CAD build for the part. Positions are in the model's coordinates, mm. A direction names the side the tool comes from. Round coordinates to 2 decimals unless told otherwise and drop trailing zeros. Loops run counter-clockwise (first coordinate to the right, second up) from the corner with the lowest first, then second, coordinate; pieces in that order, holes last. Notation, with made-up numbers: (49, 59) - (67, 59) arc R18 cw to (67, 77) - close; hole circle Ø1 at (8, 67). An arc over 180 degrees is marked (long way). One line per question, with ' | ' between items.
```python
from build123d import *

# Parameters (mm, degrees)
SKETCH_1_W          = 10
SKETCH_1_H          = 10
EXTRUDE_1_DEPTH     = 45
SKETCH_2_W          = 3
SKETCH_2_H          = 5
CUT_EXTRUDE_1_DEPTH = 7
CUT_EXTRUDE_2_REACH = 49.17
SKETCH_3_R          = 1.75


with BuildPart() as part:
    # 草图1 → 凸台-拉伸1 (new body)
    with BuildSketch(Plane.XY):
        with Locations((5, -5)):
            Rectangle(SKETCH_1_W, SKETCH_1_H)
    extrude(amount=EXTRUDE_1_DEPTH)

    # 草图2 → 切除-拉伸1 (cut)
    with BuildSketch(Plane(origin=(0, 0, 0), x_dir=(-1, 0, 0), z_dir=(0, 0, -1))):
        with Locations((-5, -5)):
            Rectangle(SKETCH_2_W, SKETCH_2_H)
    extrude(amount=-CUT_EXTRUDE_1_DEPTH, mode=Mode.SUBTRACT)

    # 草图3 → 切除-拉伸2 (cut, up to next)
    with BuildSketch(Plane(origin=(10, 0, 0), x_dir=(0, 0, -1), z_dir=(1, 0, 0)), mode=Mode.PRIVATE) as cut_extrude_2_sk1:
        with Locations(Location((-3.5, -5, 0), (0, 0, 90))):
            Circle(SKETCH_3_R)
    cut_extrude_2_tool1 = extrude(cut_extrude_2_sk1.sketch, amount=-CUT_EXTRUDE_2_REACH, mode=Mode.PRIVATE) & part.part
    add(cut_extrude_2_tool1.solids().sort_by_distance((10, -5, 3.5))[0], mode=Mode.SUBTRACT)


solid = part.part
```
(1) Drop a flat-ended pin along its axis: P1, Ø1.5, axis at x = 4.5, y = -5, coming from the -Z side. Give the stop position or say it passes through.
Results found:
P1: stops at z = 7
(2) Probe L1, parallel to Z at x = 8.75, y = -5; L2, parallel to Z at x = 4.5, y = -4.75; L3, parallel to Z at x = 7.5, y = -4. List the from-to ranges inside material, lowest first.
Results found:
L1: z = 0 to 1.75, 5.25 to 45 | L2: z = 7 to 45 | L3: z = 0 to 2.06, 4.94 to 45
(3) Tool access for faces 1 (the face through (5, -5, 7)), 2 (the face through (5, -10, 22)): list every direction of +Z, -Z, +X, -X, +Y, -Y with a clear straight run to the whole face (end or side of a thin tool).
Results found:
face 1: -Z | face 2: +Z, -Z, +X, -X, -Y
(4) Cut at A-A, the plane y = -5. Write the cut outline in (x, z), then the cut area to 3 significant figures.
Results found:
outline: (0, 0) - (3.5, 0) - (3.5, 7) - (6.5, 7) - (6.5, 5.25) - (10, 5.25) - (10, 45) - (0, 45) - close; (6.5, 0) - (10, 0) - (10, 1.75) - (6.5, 1.75) - close | area: 417 mm²
(5) Cut at B-B, the plane z = 6. Write the cut outline in (x, y), then the cut area to 3 significant figures.
Results found:
outline: (0, -10) - (10, -10) - (10, 0) - (0, 0) - close; hole (3.5, -7.5) - (6.5, -7.5) - (6.5, -2.5) - (3.5, -2.5) - close | area: 85.0 mm²
(6) Two-plate mould, pull along Z, no slides. Class faces 3 (the face through (5, -7.5, 3)), 4 (the face through (7, -5, 0)), 5 (the face through (8.27, -6.39, 2.44)): released by +Z, released by -Z, zero draft, split by the parting line, or undercut.
Results found:
face 3: zero draft | face 4: released by -Z | face 5: undercut
